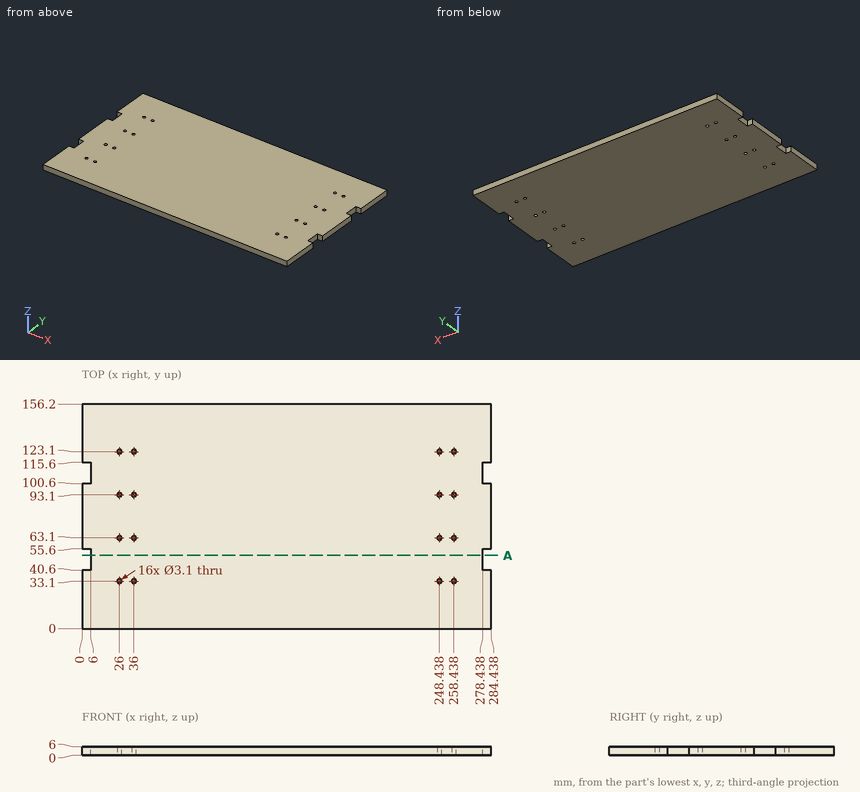
Input: dimensioned drawing with shaded views. Units: mm. Origin: part minimum x, y, z. Give positions to 0.01 mm unless a question says otherwise; leave off trailing zeros. Order: outer loops, then holes, each group sorted by start corner. A loop starts at its lowest first (then second) coordinate and runs counter-clockwise, first axis right, second up. Notation, with made-up numbers: (-24.75, 44.5) -> (31.25, 44.5) arc R19 cw to (31.25, 62.5) -> close; hole circle Ø1 at (56.5, 11.25). An arc over 180 degrees is marked (long way). Write item = value, one per line.
Item 1: Section query A-A (y = 51). Output: boundary loops of the cut face in (x, z).
Check result:
outline = (6, 0) -> (278.44, 0) -> (278.44, 6) -> (6, 6) -> close
Item 2: Contact query for flat-ended pins moving along their axis: pin 1 (3 mm diameter, centred on x = 258.438, y = 93.1, fed in from -Z); pin 2 (3 mm diameter, centred on y = 110, z = 2, fed in from +X). Output: stop coordinate, or through.
Check result:
pin_1 = through
pin_2 = 278.44
Item 3: Ray query, probe 1 along X at (y, z) = (93.1, 2.25); probe 2 along X at (y, z) = (114, 2.9). Return the intervals inside material, ascending.
Check result:
probe_1 = 0 to 24.45, 27.55 to 34.45, 37.55 to 246.89, 249.99 to 256.89, 259.99 to 284.44
probe_2 = 6 to 278.44
